from build123d import *

# Parameters (mm, degrees)
SKETCH1_R           = 10.425
SKETCH1_R_2         = 8.575
BOSS_EXTRUDE1_DEPTH = 14
SKETCH1_2_R         = 8.575
BOSS_EXTRUDE2_DEPTH = 14
SKETCH1_3_R         = 8.575
CUT_EXTRUDE1_DEPTH  = 4
CUT_EXTRUDE3_START  = 4
CUT_EXTRUDE3_DEPTH  = 4


with BuildPart() as part:
    # Sketch1 → Boss-Extrude1 (new body)
    with BuildSketch(Plane(origin=(0, 0, 0), x_dir=(1, 0, 0), z_dir=(0, 1, 0))):
        with Locations(Location((0, 0, 0), (0, 0, 270))):
            Circle(SKETCH1_R)
        with Locations(Location((0, 0, 0), (0, 0, 270))):
            Circle(SKETCH1_R_2, mode=Mode.SUBTRACT)
    extrude(amount=BOSS_EXTRUDE1_DEPTH)

    # Sketch1_2 → Boss-Extrude2 (add)
    with BuildSketch(Plane(origin=(0, 0, 0), x_dir=(1, 0, 0), z_dir=(0, 1, 0))):
        Circle(SKETCH1_2_R)
    extrude(amount=BOSS_EXTRUDE2_DEPTH)

    # Sketch1_3 → Cut-Extrude1 (cut)
    with BuildSketch(Plane(origin=(0, 0, 0), x_dir=(1, 0, 0), z_dir=(0, 1, 0))):
        with Locations(Location((0, 0, 0), (0, 0, 270))):
            Circle(SKETCH1_3_R)
    extrude(amount=CUT_EXTRUDE1_DEPTH, mode=Mode.SUBTRACT)

    # Sketch2 → Cut-Extrude3 (cut)
    with BuildSketch(Plane.XZ.offset(-4).offset(CUT_EXTRUDE3_START)):
        with BuildLine():
            Line((-1.6, -8.424406507), (-1.6, -11.258312908))
            Line((-1.6, -11.258312908), (1.6, -11.258312908))
            Line((1.6, -11.258312908), (1.6, -8.424406507))
            ThreePointArc((1.6, -8.424406507), (0, -8.575), (-1.6, -8.424406507))
        make_face()
        with BuildLine():
            Line((-10.902270297, -1.6), (-8.424406507, -1.6))
            ThreePointArc((-8.424406507, -1.6), (-8.575, 0), (-8.424406507, 1.6))
            Line((-8.424406507, 1.6), (-10.902270297, 1.6))
            Line((-10.902270297, 1.6), (-10.902270297, -1.6))
        make_face()
        with BuildLine():
            Line((-1.6, 10.963656954), (-1.6, 8.424406507))
            ThreePointArc((-1.6, 8.424406507), (-0.803535687, 8.537268615), (0, 8.575))
            ThreePointArc((0, 8.575), (0.803535687, 8.537268615), (1.6, 8.424406507))
            Line((1.6, 8.424406507), (1.6, 10.963656954))
            Line((1.6, 10.963656954), (-1.6, 10.963656954))
        make_face()
        with BuildLine():
            ThreePointArc((8.424406507, 1.6), (8.575, 0), (8.424406507, -1.6))
            Line((8.424406507, -1.6), (11.025043611, -1.6))
            Line((11.025043611, -1.6), (11.025043611, 1.6))
            Line((11.025043611, 1.6), (8.424406507, 1.6))
        make_face()
    extrude(amount=-CUT_EXTRUDE3_DEPTH, mode=Mode.SUBTRACT)

    # Sketch4 → Revolve4 (revolve)
    with BuildSketch(Plane(origin=(0, 0, 0), x_dir=(0, 0, -1), z_dir=(1, 0, 0))):
        with BuildLine():
            Line((0.364875, 33.3), (10.425, 14))
            Line((10.425, 14), (0, 14))
            Line((0, 14), (0, 33.521277517))
            ThreePointArc((0, 33.521277517), (0.213364421, 33.461635627), (0.364875, 33.3))
        make_face()
    revolve(axis=Axis((0, 14, 0), (0, 1, 0)))


solid = part.part
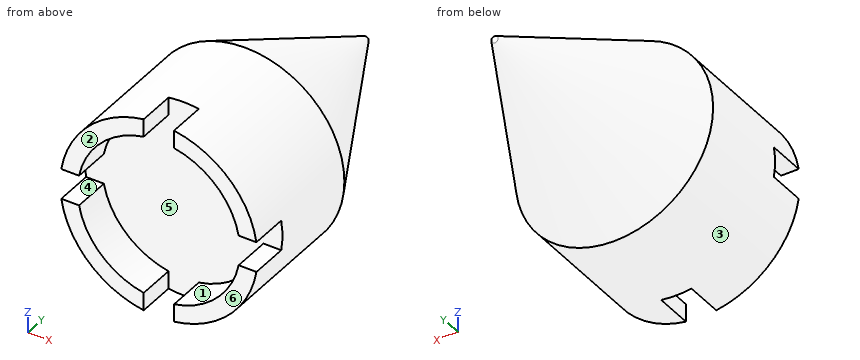
CAD build for the part. Positions are in the model's coordinates, mm. Face numbers are marked on the shaded views. A direction names the side the tool comes from. Round coordinates to 2 decimals unless told otherwise and drop trailing zeros. Order: outer loops, then holes, each group sorted by start corner. A loop starts at its lowest first (then second) coordinate and runs counter-clockwise, first axis right, second up. Notation, with made-up numbers: (81.5, 41.25) -> (104.5, 41.25) arc R34 cw to (104.5, 79.25) -> close; hole circle Ø1 at (11, 39). An arc over 180 degrees is marked (long way). Write item = value, one per line. Start each with the question number.
(1) Probe line 1 (Z direction, x = 3.5, y = 3); line 2 (X direction, y = 18, z = 4); line 3 (Y direction, x = 4.5, z = 8.75). List the from-to ranges inside material, lowest first. Write a range as [from, to].
(2) Which spindle directions (+Z, -Z, +X, -X, +Y, -Y) get a long thin tool onto all of the face, cutting with end or side? Do the marked faces 4, 5 and 6. Say none if no direction does.
(3) Pull direction X, two halves, no side cores. Call the marked faces 1, 2 and 3: released by +X, released by -X, zero draft, split by the parting line, or undercut.
(4) Pin check, flat tips, straight feed: P1, Ø5, axis at x = 1, y = 21.5, coming from the -Z side; P2, Ø3, axis at x = -1.5, y = 26, coming from the -Z side; P3, Ø0.6, axis at y = 1.5, z = 9.5, coming from the +X side. Stop position of each tip, or through.
(5) Cut at A-A, the plane z = 0. List the corners of the cut face in (x, y) (3 decimals), then the cut area to 3 significant figures.
(6) Cut at C-C, the plane x = 0. List the corners of the cut face in (y, z) (3 decimals).
(7) Cut at D-D, the plane y = 26. List the corners of the cut face in (x, z).
(8) Cut at B-B, the plane y = 12.5. List the corners of the cut face in (x, z) (3 decimals), then the cut area to 3 significant figures.
Model answer:
q1.line_1 = [-9.82, -7.83], [7.83, 9.82]
q1.line_2 = [-7.32, 7.32]
q1.line_3 = [0, 15.12]
q2.face_4 = +X, -X, -Y
q2.face_5 = -Y
q2.face_6 = +Z, -Z, +X, -X, -Y
q3.face_1 = undercut
q3.face_2 = zero draft
q3.face_3 = split by the parting line
q4.P1 = -7.78
q4.P2 = -4.8
q4.P3 = 4.9
q5.outline = (-10.425, 4) -> (10.425, 4) -> (10.425, 14) -> (0.365, 33.3) arc R0.411 ccw to (-0.365, 33.3) -> (-10.425, 14) -> close
q5.area = 417 mm2
q6.outline = (4, -10.425) -> (14, -10.425) -> (33.3, -0.365) arc R0.411 ccw to (33.3, 0.365) -> (14, 10.425) -> (4, 10.425) -> close
q7.outline = circle Ø8.34 at (0, 0)
q8.outline = circle Ø20.85 at (0, 0)
q8.area = 341 mm2
